Geometry check sheet. Reference: the model listing, model coordinates, mm. Coordinates: 2 decimals unless noted, no trailing zeros. Write each loop counter-clockwise with the first axis right and the second up, starting at its lowest first coordinate (ties: lowest second). Pieces come first, ordered by that corner, then holes. Notation, with made-up numbers: (5.5, 26) -> (9.5, 26) arc R18 ccw to (9.5, 50) -> close; hole circle Ø10 at (-12, -8). An arc over 180 degrees is marked (long way). Answer in a Markdown table with one row per item. Add a question column.
Q1. Section check B-B, the plane z = 39.5. Record the boundary of the cut face in (x, y), and give its area (3 significant figures).
Q2. Thickness scan on line 1 (Z direction, x = -162.5, y = 3.75); line 2 (Z direction, x = 132, y = -0.5); line 3 (X direction, y = 7.5, z = 38.5). Record the ranges inside material, lowest first.
Q3. Section check A-A, the plane x = -125. Count the separate pieces of the cut face and the enclosed holes in it, and give its area (3 significant figures).
Q4. Section check C-C, the plane y = 3.25. Record the boundary of the cut face in (x, z), and give its area (3 significant figures).
Q5. Gauge pin test, flat ends, axial feed: P1, Ø1, axis at x = -9.5, y = 0.5, coming from the -Z side; P2, Ø2.5, axis at y = 0, z = 65, coming from the -X side; P3, Ø5, axis at y = 6.5, z = 58.5, coming from the -X side. Record the tip position at first contact, or that the pin passes through.
```python
from build123d import *

# Parameters (mm, degrees)
SKETCH1_W           = 393.7
SKETCH1_H           = 97.79635
BOSS_EXTRUDE1_DEPTH = 1.5875
SKETCH4_W           = 393.4968
SKETCH4_H           = 97.59315
BOSS_EXTRUDE4_DEPTH = 6.35


with BuildPart() as part:
    # Sketch1 → Boss-Extrude1 (new body, symmetric)
    with BuildSketch(Plane(origin=(0, 0, 0), x_dir=(1, 0, 0), z_dir=(0, 1, 0))):
        Polygon((196.85, 55.248175), (-203.2, 55.248175), (-203.2, -55.248175), (196.85, -55.248175), (196.85, -61.648975), (-203.2, -61.648975), (-203.2, -72.3646), (190.5, -72.3646), (203.2, -72.3646), (203.2, 72.3646), (190.5, 72.3646), (-203.2, 72.3646), (-203.2, 61.648975), (196.85, 61.648975), align=None)
        Rectangle(SKETCH1_W, SKETCH1_H, mode=Mode.SUBTRACT)
    extrude(amount=BOSS_EXTRUDE1_DEPTH, both=True)

    # Sketch4 → Boss-Extrude4 (add)
    with BuildSketch(Plane(origin=(0, 1.5875, 0), x_dir=(1, 0, 0), z_dir=(0, 1, 0))):
        Polygon((-203.3016, 61.547375), (196.7484, 61.547375), (196.7484, 55.349775), (-203.3016, 55.349775), (-203.3016, -55.349775), (196.7484, -55.349775), (196.7484, -61.547375), (-203.3016, -61.547375), (-203.3016, -72.4662), (203.3016, -72.4662), (203.3016, 72.4662), (-203.3016, 72.4662), align=None)
        Rectangle(SKETCH4_W, SKETCH4_H, mode=Mode.SUBTRACT)
    extrude(amount=BOSS_EXTRUDE4_DEPTH)


solid = part.part
```
Calculated:
| question | item | result |
|---|---|---|
| 1 | outline | (-203.3, 1.59) -> (-203.2, 1.59) -> (-203.2, -1.59) -> (-196.85, -1.59) -> (-196.85, 1.59) -> (-196.75, 1.59) -> (-196.75, 7.94) -> (-203.3, 7.94) -> close; (196.75, 1.59) -> (196.85, 1.59) -> (196.85, -1.59) -> (203.2, -1.59) -> (203.2, 1.59) -> (203.3, 1.59) -> (203.3, 7.94) -> (196.75, 7.94) -> close |
| 1 | area | 124 mm² |
| 2 | line 1 | z = -72.47 to -61.55, -55.35 to -48.8, 48.8 to 55.35, 61.55 to 72.47 |
| 2 | line 2 | z = -72.36 to -61.65, -55.25 to -48.9, 48.9 to 55.25, 61.65 to 72.36 |
| 2 | line 3 | x = -203.3 to -196.75, 196.75 to 203.3 |
| 3 | separate pieces | 4 |
| 3 | enclosed holes | 0 |
| 3 | area | 330 mm² |
| 4 | outline | (-203.3, -72.47) -> (203.3, -72.47) -> (203.3, 72.47) -> (-203.3, 72.47) -> (-203.3, 61.55) -> (196.75, 61.55) -> (196.75, 55.35) -> (-203.3, 55.35) -> (-203.3, -55.35) -> (196.75, -55.35) -> (196.75, -61.55) -> (-203.3, -61.55) -> close; hole (-196.75, -48.8) -> (196.75, -48.8) -> (196.75, 48.8) -> (-196.75, 48.8) -> close |
| 4 | area | 15,600 mm² |
| 5 | P1 | stops at z = -72.36 |
| 5 | P2 | stops at x = -203.2 |
| 5 | P3 | stops at x = 196.75 |
